Part model, mm, in its own coordinate system. Give positions to 0.01 mm unless a question says otherwise; leave off trailing zeros. Loops run counter-clockwise (first coordinate to the right, second up) from the corner with the lowest first, then second, coordinate; pieces in that order, holes last. Notation, with made-up numbers: (-8, 86) -> (49, 86) arc R23 cw to (49, 116) -> close; hole circle Ø2 at (26.25, -15.75). An arc over 180 degrees is marked (long way). One line per question, with ' | ' between items.
```python
from build123d import *

# Parameters (mm, degrees)
CROQUIS1_W              = 20
CROQUIS1_H              = 10.000326638
CROQUIS1_R              = 1.625
SALIENTE_EXTRUIR1_DEPTH = 4
REDONDEO1_R             = 3


with BuildPart() as part:
    # Croquis1 → Saliente-Extruir1 (new body)
    with BuildSketch(Plane.XY):
        Rectangle(CROQUIS1_W, CROQUIS1_H)
        with Locations((-6, 0)):
            Circle(CROQUIS1_R, mode=Mode.SUBTRACT)
        with Locations((6, 0)):
            Circle(CROQUIS1_R, mode=Mode.SUBTRACT)
    extrude(amount=SALIENTE_EXTRUIR1_DEPTH)

    # Redondeo1
    redondeo1_edges = [part.edges().sort_by_distance(p)[0] for p in [
        (10, -5.000163319, 2),
        (-10, -5.000163319, 2),
        (-10, 5.000163319, 2),
        (10, 5.000163319, 2),
    ]]
    fillet(redondeo1_edges, radius=REDONDEO1_R)


solid = part.part
```
1) Saw through at B-B (z = 2.85). Give the cut face in (x, y) (3 decimals).
Found:
outline: (-10, -2) arc R3 ccw to (-7, -5) -> (7, -5) arc R3 ccw to (10, -2) -> (10, 2) arc R3 ccw to (7, 5) -> (-7, 5) arc R3 ccw to (-10, 2) -> close; hole circle Ø3.25 at (-6, 0); hole circle Ø3.25 at (6, 0)
2) Saw through at A-A (y = 0). Give the cut face in (x, z) (3 decimals), and give its area (3 significant figures).
Found:
outline: (-10, 0) -> (-7.625, 0) -> (-7.625, 4) -> (-10, 4) -> close; (-4.375, 0) -> (4.375, 0) -> (4.375, 4) -> (-4.375, 4) -> close; (7.625, 0) -> (10, 0) -> (10, 4) -> (7.625, 4) -> close | area: 54.0 mm2
3) Pull direction Y, two halves, no side cores. Call faces 1 (the cylindrical face through (9.1, -4.14, 2.03)), 2 (the cylindrical face through (4.377, 0.071, 1.972)), 3 (the cylindrical face through (9.1, 4.14, 2.03)): pulls with the +Y half, pulls with the -Y half, needs draft (parallel to the pull), parting line crosses it, or undercut.
Found:
face 1: pulls with the -Y half | face 2: undercut | face 3: pulls with the +Y half
4) Saw through at D-D (x = 8). Give the cut face in (y, z), and give its area (3 significant figures).
Found:
outline: (-4.83, 0) -> (4.83, 0) -> (4.83, 4) -> (-4.83, 4) -> close | area: 38.6 mm2
5) Drill centre lines: line 1 (Y direction, x = -6, z = 3) (3 decimals); line 2 (X direction, y = -0.25, z = 1.4); line 3 (Y direction, x = 5.5, z = 2.25). Where is each one in solid material? Low to high.
Found:
line 1: -5 to -1.625, 1.625 to 5 | line 2: -10 to -7.61, -4.39 to 4.39, 7.61 to 10 | line 3: -5 to -1.55, 1.55 to 5
6) Pin check, flat tips, straight feed: P1, Ø5, axis at x = -7.5, y = 0.5, coming from the +Z side; P2, Ø1.5, axis at y = -3, z = 3, coming from the -X side. Stop position of each tip, or through.
Found:
P1: z = 4 | P2: x = -9.99
7) Saw through at C-C (x = -5.25). Give the cut face in (y, z).
Found:
outline: (-5, 0) -> (-1.44, 0) -> (-1.44, 4) -> (-5, 4) -> close; (1.44, 0) -> (5, 0) -> (5, 4) -> (1.44, 4) -> close
